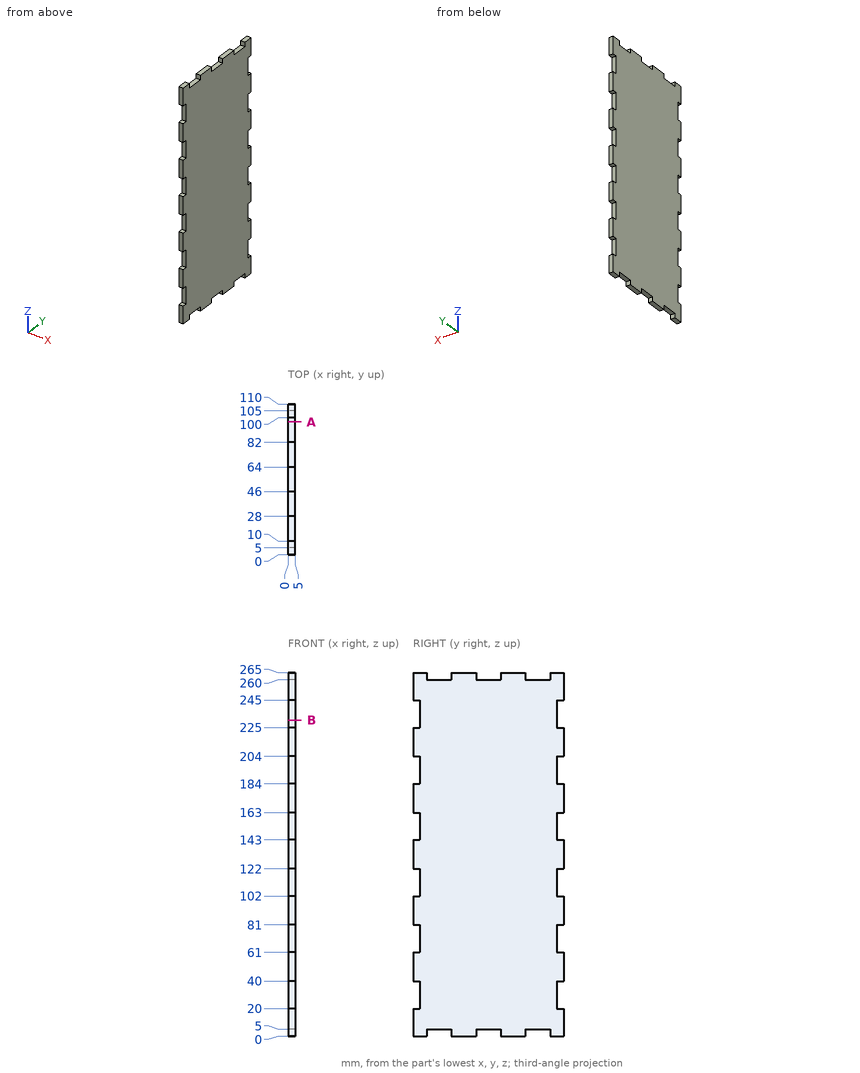
Check sheet for the drawn part. Datum: minimum x, y, z corner. Units: mm. Round coordinates to 2 decimals unless told otherwise and drop trailing zeros. Order: outer loops, then holes, each group sorted by start corner. A loop starts at its lowest first (then second) coordinate and runs counter-clockwise, first axis right, second up. Notation, with made-up numbers: (72, 8) -> (103, 8) arc R32 ccw to (103, 39) -> close; hole circle Ø7 at (66, -4.5). An arc over 180 degrees is marked (long way). Return JSON: item names as keys, results as strings. Group by question number.
Q1. Section check A-A, the plane y = 97. Record the boundary of the cut face in (x, z), plus the area to 4 significant figures.
Q2. Gauge pin test, flat ends, axial feed: pin 1 (2.5 mm diameter, centred on x = 2.5, y = 14.5, fed in from -Z); pin 2 (1.5 mm diameter, centred on x = 3.5, y = 87.5, fed in from +Z). Record the tip position at first contact, or that the pin passes through.
Q3. Material ranges on probe 1 along Z at (x, y) = (4.6, 84.5); probe 2 along Y at (x, z) = (3.8, 21.5), recorded low to high. Write a range as from..to.
Q4. Section check B-B, the plane z = 230.5. Record the boundary of the cut face in (x, y), plus the area to 3 significant figures.
Numbers:
{
 "1": {"outline": "(0, 5) -> (5, 5) -> (5, 260) -> (0, 260) -> close", "area": "1,275 mm^2"},
 "2": {"pin 1": "z = 5", "pin 2": "z = 260"},
 "3": {"probe 1": "5..260", "probe 2": "5..105"},
 "4": {"outline": "(0, 5) -> (5, 5) -> (5, 105) -> (0, 105) -> close", "area": "500 mm^2"}
}
